Source: CAD feature listing. Evaluate the final solid. Frame: model axes, mm. A direction names the side the tool comes from. Round coordinates to 2 decimals unless told otherwise and drop trailing zeros. Write each loop counter-clockwise with the first axis right and the second up, starting at its lowest first coordinate (ties: lowest second). Pieces come first, ordered by that corner, then holes.
Autodesk Inventor part; units mm, degrees
ref_plane "Work Plane16" through (0, 0, 0) normal (1, 0, 0) x (0, 1, 0)
ref_plane "Work Plane17" through (0, 0, 0) normal (0, -1, 0) x (1, 0, 0)
ref_plane "YZ Plane" through (0, 0, 0) normal (1, 0, 0) x (0, 1, 0)
sketch "Sketch18" plane through (0, 0, 0) normal (0, 0, 1) x (1, 0, 0)
  circle A0 centre (0, 0) radius 20.3835
  dimension "d50" = 40.767
extrude "Extrusion10" add sketch "Sketch18" against normal blind 50.8
sketch "Sketch24" plane through (0, 0, 0) normal (0, 0, 1) x (1, 0, 0)
  line L0 (0, 0) -> (20.3835, 0)
  circle A0 centre (0, 0) radius 20.3835
  line L1 (0, 0) -> (0, 20.3835)
ref_plane "Work Plane16" through (0, 0, 0) normal (1, 0, 0) x (0, 1, 0)
ref_plane "Work Plane17" through (0, 0, 0) normal (0, -1, 0) x (1, 0, 0)
sketch "Sketch25" plane through (0, 0, 0) normal (1, 0, 0) x (0, 1, 0)
  line L0 (-20.3835, -50.8) -> (20.3835, -50.8)
  circle A0 centre (0, -50.8) radius 20.3835
  point P0 (0, 0)
  dimension "d67" = 40.767
sketch "Sketch26" plane through (0, 0, 0) normal (0, -1, 0) x (1, 0, 0)
  line L0 (-20.3835, -50.8) -> (20.3835, -50.8)
  circle A0 centre (0, -50.8) radius 20.3835
  point P0 (0, 0)
extrude "Extrusion14" add sketch "Sketch26" against normal blind 50.8
extrude "Extrusion15" add sketch "Sketch25" along normal blind 50.8
sketch "Sketch27" plane through (0, 0, 0) normal (-1, 0, 0) x (0, 0, 1)
  line L0 (-50.8, 0) -> (-50.8, -20.3835)
  line L1 (-50.8, 0) -> (-50.8, -20.3835)
  circle A0 centre (-50.8, 0) radius 20.3835
  line L2 (-50.8, 0) -> (-71.1835, 0)
  line L3 (-50.8, 0) -> (-71.1835, 0)
  arc A1 (-71.1835, 0) -> (-50.8, -20.3835) centre (-50.8, 0) ccw
  point P0 (0, 0)
revolve "Revolution12" add sketch "Sketch27" angle 90 about axis through (0, 0, -50.8) along (0, 1, 0) picked at (-52.3119, -13.4186) contours L0 A0 L2
sketch "Sketch28" plane through (0, 0, 0) normal (0, 0, 1) x (1, 0, 0)
  line L0 (20.3835, 20.3835) -> (0, 0)
  circle A0 centre (0, 0) radius 12.7
  line L1 (0, 0) -> (0, -20.3835)
  circle A1 centre (0, 0) radius 16.7767
  point P0 (14.4133, 14.4133)
  dimension "d73" = 25.4
  dimension "d74" = 33.5534
sketch "Sketch29" plane through (0, 50.8, -50.8) normal (0, 1, 0) x (1, 0, 0)
  line L0 (0, 20.3835) -> (0, 0)
  circle A0 centre (0, 0) radius 12.7
  line L1 (0, 0) -> (-20.3835, 0)
  circle A1 centre (0, 0) radius 16.7767
  point P0 (0, -50.8)
  dimension "d75" = 25.4
  dimension "d76" = 33.5534
sketch "Sketch30" plane through (50.8, 0, -50.8) normal (1, 0, 0) x (0, 0, -1)
  circle A0 centre (0, 0) radius 20.3835
  circle A1 centre (0, 0) radius 12.7
  line L0 (-20.3835, 20.3835) -> (0, 0)
  circle A2 centre (0, 0) radius 16.7767
  point P0 (-50.8, 0)
  point P1 (-14.4133, 14.4133)
  dimension "d77" = 25.4
  dimension "d78" = 33.5534
extrude "Extrusion16" cut sketch "Sketch30" against normal blind 50.8 contours A1
extrude "Extrusion17" cut sketch "Sketch28" against normal blind 50.8 contours A0 L1 L0 | L0 L1 A0
extrude "Extrusion18" cut sketch "Sketch29" against normal blind 50.8 contours A0 L1 L0 | L0 L1 A0
extrude "Extrusion19" cut sketch "Sketch30" against normal blind 31.75 contours A2
extrude "Extrusion20" cut sketch "Sketch28" against normal blind 31.75 contours A1 L1 A0 L0 | L0 A0 L1 A1
extrude "Extrusion21" cut sketch "Sketch29" against normal blind 31.75 contours A1 L1 A0 L0 | L0 A0 L1 A1
sketch "Sketch31" plane through (0, 0, -50.8) normal (1, 0, 0) x (0, 0, -1)
  line L0 (12.7, 0) -> (0, 0)
  line L1 (0, 0) -> (0, -12.7)
  arc A0 (0, -12.7) -> (12.7, 0) centre (0, 0) ccw
  point P0 (-50.8, 0)
revolve "Revolution13" cut sketch "Sketch31" angle 90 about axis through (0, 0, -50.8) along (0, 1, 0)
properties part number "3-way 90 1 Inch"
1) Reachability of faces 1 (the face through (-16.18, -12.4, -19.4)), 2 (the face through (35.15, 5.04, -66.8)), 3 (the face through (-9.36, 11.775, -59.383)), 4 (the face through (-17, 50.8, -54)) from +Z, -Z, +X, -X, +Y, -Y: full face, straight path, thin tool, end or side. Return the list, or none.
Taken from the geometry:
face 1: +Z
face 2: +X
face 3: +Y
face 4: +Z, -Z, +X, -X, +Y
2) Section query A-A on y = -3. Return the cut outline in (x, z), then the cut area to 3 significant figures.
Taken from the geometry:
outline: (-20.16, -50.8) arc R20.16 ccw to (0, -70.96) - (50.8, -70.96) - (50.8, -67.31) - (19.05, -67.31) - (19.05, -63.14) - (0, -63.14) arc R12.34 cw to (-12.34, -50.8) - (-12.34, -31.75) - (-16.51, -31.75) - (-16.51, 0) - (-20.16, 0) - close; (12.34, -38.46) - (19.05, -38.46) - (19.05, -34.29) - (50.8, -34.29) - (50.8, -30.64) - (20.16, -30.64) - (20.16, 0) - (16.51, 0) - (16.51, -31.75) - (12.34, -31.75) - close
area: 1,010 mm2
3) Contact query for flat-ended pins moving along their axis: P1, Ø3, axis at x = 2.5, y = 42, coming from the -Z side; P2, Ø10, axis at x = 1, y = -8, coming from the -Z side; P3, Ø15, axis at x = 0, z = -50.8, coming from the +Y side. Output: stop coordinate, or through.
Taken from the geometry:
P1: stops at z = -71.16
P2: stops at z = -70.96
P3: stops at y = -10.25
4) Pull-direction query (X, two-part tool) for faces 5 (the face through (-16.18, 30.69, -63.2)), 6 (the face through (50.8, -17, -54)), 7 (the face through (-3, 13, -31.75)); classes: released by +X, released by -X, zero draft, split by the parting line, or undercut.
Taken from the geometry:
face 5: split by the parting line
face 6: released by +X
face 7: undercut
5) Material intervals for line 1 (Y direction, x = 0, z = -17.5); line 2 (X direction, y = 13.75, z = -50.8); line 3 (Z direction, x = 34, y = 0), sorted ascending.
Taken from the geometry:
line 1: y = -20.38 to -16.78, 16.78 to 20.38
line 2: x = -20.38 to -12.7, 12.7 to 19.05
line 3: z = -71.18 to -67.58, -34.02 to -30.42
6) Section query C-C on x = 43.5. Return the cut outline in (y, z).
Taken from the geometry:
outline: circle Ø40.77 at (0, -50.8); hole circle Ø33.55 at (0, -50.8)
7) Section query B-B on z = -55. Return the cut outline in (x, y), then the cut area to 3 significant figures.
Taken from the geometry:
outline: (-19.95, 0) arc R19.95 ccw to (0, -19.95) - (50.8, -19.95) - (50.8, -16.24) - (19.05, -16.24) - (19.05, -11.99) - (0, -11.99) arc R11.99 cw to (-11.99, 0) - (-11.99, 19.05) - (-16.24, 19.05) - (-16.24, 50.8) - (-19.95, 50.8) - close; (11.99, 11.99) - (19.05, 11.99) - (19.05, 16.24) - (50.8, 16.24) - (50.8, 19.95) - (19.95, 19.95) - (19.95, 50.8) - (16.24, 50.8) - (16.24, 19.05) - (11.99, 19.05) - close
area: 1,020 mm2
